Could you check a few things on this model? Use its own coordinates, in mm. A direction names the side the tool comes from. Coordinates: 2 decimals unless noted, no trailing zeros. Loops run counter-clockwise (first coordinate to the right, second up) from the corner with the lowest first, then second, coordinate; pieces in that order, holes last. Notation, with made-up numbers: (14, -21.75) - (41, -21.75) arc R7 cw to (41, -17.75) - close; hole circle Ø5 at (27.5, 85). An arc over 180 degrees is marked (long way). Use CSV: the item, a comma, the result in double quotes.
from build123d import *

# Parameters (mm, degrees)
SKETCH1_W                                        = 38.1
SKETCH1_H                                        = 19.05
EXTRUDE1_DEPTH                                   = 69.85
CUT_EXTRUDE1_REACH                               = 21.05
SKETCH2_R                                        = 9.525
CSK_FOR_M10_FLAT_HEAD_MACHINE_SCREW1_D           = 11
CSK_FOR_M10_FLAT_HEAD_MACHINE_SCREW1_DEPTH       = 29.464
CSK_FOR_M10_FLAT_HEAD_MACHINE_SCREW1_CSINK_D     = 20
CSK_FOR_M10_FLAT_HEAD_MACHINE_SCREW1_CSINK_ANGLE = 90
CSK_FOR_M10_FLAT_HEAD_MACHINE_SCREW1_TIP         = 3.304733405
SKETCH5_R                                        = 15.9385
CUT_EXTRUDE2_DEPTH                               = 12.7
BOSS_EXTRUDE1_DEPTH                              = 12.7


with BuildPart() as part:
    # Sketch1 → Extrude1 (new body, symmetric)
    with BuildSketch(Plane.XY):
        Rectangle(SKETCH1_W, SKETCH1_H)
    extrude(amount=EXTRUDE1_DEPTH, both=True)

    # Sketch2 → Cut-Extrude1 (cut, up to next)
    with BuildSketch(Plane(origin=(0, 9.525, 0), x_dir=(1, 0, 0), z_dir=(0, 1, 0)), mode=Mode.PRIVATE) as cut_extrude1_sk1:
        with Locations((0, 47.625)):
            Circle(SKETCH2_R)
    cut_extrude1_tool1 = extrude(cut_extrude1_sk1.sketch, amount=-CUT_EXTRUDE1_REACH, mode=Mode.PRIVATE) & part.part
    add(cut_extrude1_tool1.solids().sort_by_distance((0, 9.525, -47.625))[0], mode=Mode.SUBTRACT)
    # Sketch2 → Cut-Extrude1 (cut, up to next)
    with BuildSketch(Plane(origin=(0, 9.525, 0), x_dir=(1, 0, 0), z_dir=(0, 1, 0)), mode=Mode.PRIVATE) as cut_extrude1_sk2:
        with Locations((0, -47.625)):
            Circle(SKETCH2_R)
    cut_extrude1_tool2 = extrude(cut_extrude1_sk2.sketch, amount=-CUT_EXTRUDE1_REACH, mode=Mode.PRIVATE) & part.part
    add(cut_extrude1_tool2.solids().sort_by_distance((0, 9.525, 47.625))[0], mode=Mode.SUBTRACT)

    # CSK for M10 Flat Head Machine Screw1
    with Locations(Plane(origin=(0, 9.525, 0), x_dir=(-1, 0, 0), z_dir=(0, 1, 0))):
        with Locations((0, 0)):
            CounterSinkHole(CSK_FOR_M10_FLAT_HEAD_MACHINE_SCREW1_D / 2, CSK_FOR_M10_FLAT_HEAD_MACHINE_SCREW1_CSINK_D / 2, depth=CSK_FOR_M10_FLAT_HEAD_MACHINE_SCREW1_DEPTH, counter_sink_angle=CSK_FOR_M10_FLAT_HEAD_MACHINE_SCREW1_CSINK_ANGLE)
            with Locations((0, 0, -(CSK_FOR_M10_FLAT_HEAD_MACHINE_SCREW1_DEPTH + CSK_FOR_M10_FLAT_HEAD_MACHINE_SCREW1_TIP / 2))):  # 118° drill point
                Cone(0, CSK_FOR_M10_FLAT_HEAD_MACHINE_SCREW1_D / 2, CSK_FOR_M10_FLAT_HEAD_MACHINE_SCREW1_TIP, mode=Mode.SUBTRACT)

    # Sketch5 → Cut-Extrude2 (cut)
    with BuildSketch(Plane.XZ.offset(9.525)):
        Circle(SKETCH5_R)
    extrude(amount=-CUT_EXTRUDE2_DEPTH, mode=Mode.SUBTRACT)

    # Sketch6 → Boss-Extrude1 (add)
    with BuildSketch(Plane.XZ.offset(9.525)):
        with BuildLine():
            Line((-12.7635, 9.5461432), (-12.7635, -9.5461432))
            ThreePointArc((-12.7635, -9.5461432), (-15.9385, 0), (-12.7635, 9.5461432))
        make_face()
        with BuildLine():
            Line((12.7635, 9.5461432), (12.7635, -9.5461432))
            ThreePointArc((12.7635, -9.5461432), (15.9385, 0), (12.7635, 9.5461432))
        make_face()
    extrude(amount=-BOSS_EXTRUDE1_DEPTH)


solid = part.part
(1) Thinking about a two-plate mould opening in Z: for faces 1 (the face through (0, 0, -69.85)), 2 (the face through (0, 0, 69.85)), 3 (the face through (-12.764, -3, 0)), 4 (the face through (19.05, 0, 1)), which applies, +Z half, -Z half, draft (parallel to the pull), parting line (faces both ways), or undercut?
Computed:
face 1,"-Z half"
face 2,"+Z half"
face 3,"undercut"
face 4,"draft"
(2) Please list where these lines run through material, in increasing order: line 1 (Z direction, x = 0, y = 4.4); line 2 (Z direction, x = 4.5, y = 7); line 3 (X direction, y = 4, z = 0).
Computed:
line 1,"z = -69.85 to -57.15, -38.1 to -5.5, 5.5 to 38.1, 57.15 to 69.85"
line 2,"z = -69.85 to -56.02, -39.23 to -5.97, 5.97 to 39.23, 56.02 to 69.85"
line 3,"x = -19.05 to -5.5, 5.5 to 19.05"
(3) Suppose I cut it at A-A (x = 0). State how many separate pieces and enclosed holes the cut face has, plus the area to 3 significant figures.
Computed:
separate pieces,"4"
enclosed holes,"0"
area,"1,440 mm²"
(4) Suppose I cut it at D-D (z = 40). Write out the boundary of the cut face in (x, y) (3 decimals).
Computed:
outline,"(-19.05, -9.525) - (-5.708, -9.525) - (-5.708, 9.525) - (-19.05, 9.525) - close; (5.708, -9.525) - (19.05, -9.525) - (19.05, 9.525) - (5.708, 9.525) - close"
(5) Which directions (+Z, -Z, +X, -X, +Y, -Y) give clear straight access to the entire face, cutting with the end or side of a thin tool? Please do faces 5 (the face through (-0.207, -3.264, -15.937)), 6 (the face through (-2.065, 0.133, -38.327)).
Computed:
face 5,"-Y"
face 6,"+Y, -Y"
